Answer from the drawing. Dimensions are ordinates in mm from the lowest x, y and z of the part. A direction names the side the tool comes from. Give positions to 0.01 mm unless a question says otherwise; leave off trailing zeros. Write each loop counter-clockwise with the first axis right and the second up, starting at its lowest first coordinate (ties: lowest second). Pieces come first, ordered by that corner, then holes. Notation, with made-up numbers: (88.25, 49) -> (126.25, 49) arc R25 cw to (126.25, 83) -> close; hole circle Ø11 at (26.5, 18). An arc over 180 degrees is marked (long way). Put each result on its own line as item: value. Start each with the question number.
1) A cutting plane is placed at B-B (y = 19.05). Write down the section's boundary in (x, z) (3 decimals), then the cut area to 3 significant figures.
2) A flat-ended cylindrical pin translates along its axis: pin 1 Ø10 at (x, y) = (34, 31) entering from -Z (3 decimals). Find the tip coordinate at first contact, or state that the pin passes through.
3) For the marked faces 1 and 2, determine the directions among +Z, -Z, +X, -X, +Y, -Y from which every point of the face is accessible in a straight line to the end or side of a thin tool.
4) A cutting plane is placed at D-D (z = 23). Write down the section's boundary in (x, y) (3 decimals).
5) For a pull along X with two mould halves and no side action, classify the marked faces 3, 4 and 5 as released by +X, released by -X, zero draft, split by the parting line, or undercut.
6) A cutting plane is placed at A-A (z = 19.05). Write down the section's boundary in (x, y) (3 decimals).
7) A cutting plane is placed at C-C (x = 42.5). Write down the section's boundary in (y, z) (3 decimals), then the cut area to 3 significant figures.
8) Find the intervals of material crossed by line 1 along X through (y, z) = (12.5, 19) (3 decimals); line 2 along Y through (x, z) = (1.05, 19.05), in increasing order. Write a range as from..to.
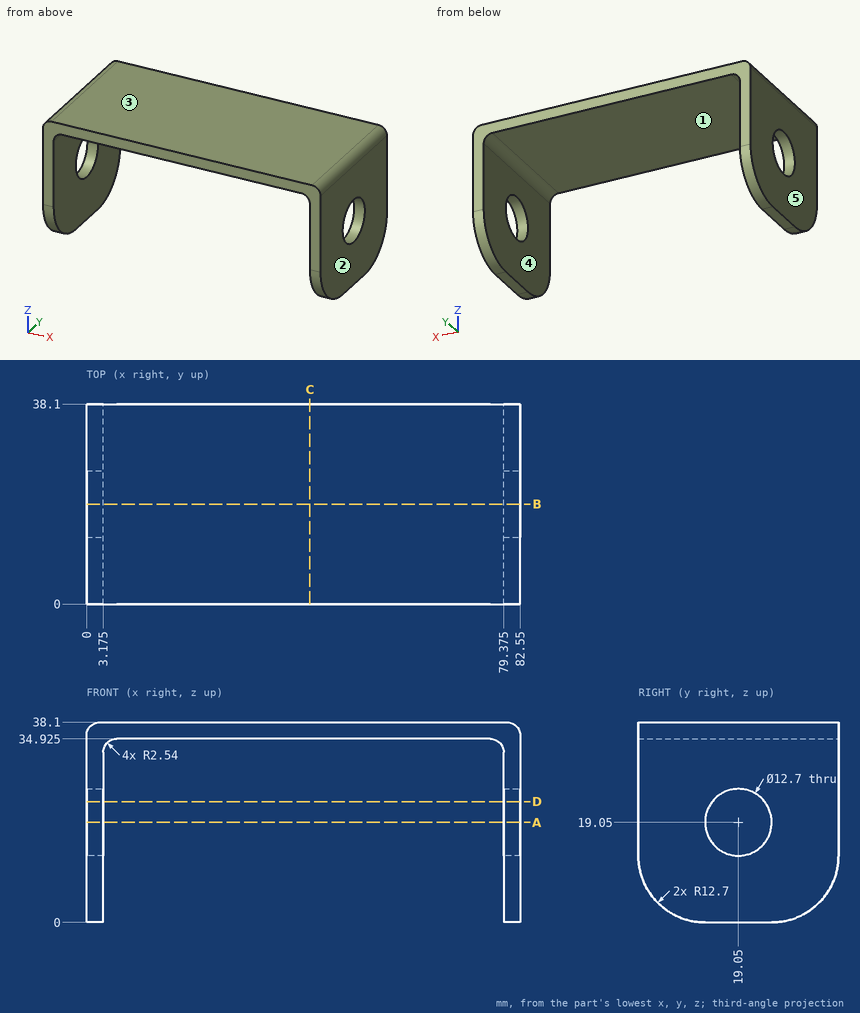
Reply:
1. outline: (0, 0) -> (3.175, 0) -> (3.175, 12.7) -> (0, 12.7) -> close; (0, 25.4) -> (3.175, 25.4) -> (3.175, 32.385) arc R2.54 cw to (5.715, 34.925) -> (76.835, 34.925) arc R2.54 cw to (79.375, 32.385) -> (79.375, 25.4) -> (82.55, 25.4) -> (82.55, 35.56) arc R2.54 ccw to (80.01, 38.1) -> (2.54, 38.1) arc R2.54 ccw to (0, 35.56) -> close; (79.375, 0) -> (82.55, 0) -> (82.55, 12.7) -> (79.375, 12.7) -> close
1. area: 403 mm2
2. pin 1: stops at z = 34.925
3. face 1: -Z, +Y, -Y
3. face 2: +Z, -Z, +X, +Y, -Y
4. outline: (0, 0) -> (3.175, 0) -> (3.175, 14.078) -> (0, 14.078) -> close; (0, 24.022) -> (3.175, 24.022) -> (3.175, 38.1) -> (0, 38.1) -> close; (79.375, 0) -> (82.55, 0) -> (82.55, 14.078) -> (79.375, 14.078) -> close; (79.375, 24.022) -> (82.55, 24.022) -> (82.55, 38.1) -> (79.375, 38.1) -> close
5. face 3: zero draft
5. face 4: undercut
5. face 5: released by -X
6. outline: (0, 0) -> (3.175, 0) -> (3.175, 12.7) -> (0, 12.7) -> close; (0, 25.4) -> (3.175, 25.4) -> (3.175, 38.1) -> (0, 38.1) -> close; (79.375, 0) -> (82.55, 0) -> (82.55, 12.7) -> (79.375, 12.7) -> close; (79.375, 25.4) -> (82.55, 25.4) -> (82.55, 38.1) -> (79.375, 38.1) -> close
7. outline: (0, 34.925) -> (38.1, 34.925) -> (38.1, 38.1) -> (0, 38.1) -> close
7. area: 121 mm2
8. line 1: x = 0..3.175, 79.375..82.55
8. line 2: y = 0..12.7, 25.4..38.1
